Autodesk Inventor part; units mm, degrees
ref_plane "YZ Plane" through (0, 0, 0) normal (1, 0, 0) x (0, 1, 0)
ref_plane "XZ Plane" through (0, 0, 0) normal (0, 1, 0) x (-1, 0, 0)
ref_plane "XY Plane" through (0, 0, 0) normal (0, 0, 1) x (1, 0, 0)
sketch "Base" plane through (0, 0, 0) normal (0, 0, 1) x (1, 0, 0)
  line L0 (0, 0) -> (-33.5334, -57.9479)
  line L1 (22.7363, 2.3748) -> (0, 0)
  line L2 (68.7163, -13.2577) -> (22.7363, 2.3748)
  line L3 (-33.5334, -57.9479) -> (-26.9158, -67.5067)
  line L4 (-26.9158, -67.5067) -> (-51.547, -128.5125)
  line L5 (-51.547, -128.5125) -> (-33.4114, -135.8348)
  line L6 (-26.9158, -67.5067) -> (12.6221, -101.6388) construction
  line L7 (12.6221, -101.6388) -> (22.7363, -101.0656)
  line L8 (12.6221, -101.6388) -> (-8.1441, -124.1457)
  line L9 (-33.4114, -135.8348) -> (-8.1441, -124.1457)
  line L10 (22.7363, 2.3748) -> (68.7163, -13.2577)
  line L11 (68.7163, -13.2577) -> (112.7039, -111.8391)
  line L12 (22.7363, 2.3748) -> (22.7363, -101.0656) construction
  line L13 (22.7363, -101.0656) -> (65.9464, -171.4033)
  line L14 (112.7039, -111.8391) -> (105.2475, -122.1197)
  line L15 (22.7363, -101.0656) -> (112.7039, -111.8391) construction
  line L16 (105.2475, -122.1197) -> (103.571, -134.8197)
  line L17 (103.571, -134.8197) -> (108.4402, -146.5492)
  line L18 (65.9464, -171.4033) -> (74.9694, -180.3406)
  line L19 (108.4402, -146.5492) -> (74.9694, -180.3406)
  circle A0 centre (85.3652, -157.1655) radius 25.4
  line L20 (-42.4792, -132.1736) -> (22.7363, -49.3454) construction
  line L21 (-33.0514, -120.1997) -> (-25.1949, -110.2215) construction
  line L22 (-35.546, -118.2356) -> (-27.6895, -108.2573)
  line L23 (-22.7004, -112.1856) -> (-30.5568, -122.1638)
  arc A1 (-35.546, -118.2356) -> (-30.5568, -122.1638) centre (-33.0514, -120.1997) ccw
  arc A2 (-22.7004, -112.1856) -> (-27.6895, -108.2573) centre (-25.1949, -110.2215) ccw
  circle A3 centre (85.3652, -157.1655) radius 4
  line L24 (0, -219.5535) -> (0, 39.3628)
  point P0 (-29.1232, -115.2106)
  point P1 (60.5618, -162.6381)
  dimension "d4" = 50.8
  dimension "d5" = 22.86
  dimension "d6" = 155.26
  dimension "d7" = 126.02
  dimension "d8" = 48.5647
  dimension "d9" = 66.9511
  dimension "d10" = 132.824
  dimension "d11" = 107.95
  dimension "d12" = 115.248
  dimension "d13" = 11.6259
  dimension "d14" = 65.7906
  dimension "d15" = 19.558
  dimension "d16" = 120
  dimension "d17" = 12.7
  dimension "d18" = 12.7
  dimension "d19" = 12.7
  dimension "d20" = 82.55
  dimension "d21" = 12.7
  dimension "d24" = 15.24
  dimension "d26" = 12.7
  dimension "d31" = 8
  dimension "d32" = 95.963
  dimension "d33" = 38.215
  dimension "d34" = 22.545
  dimension "d35" = 7.52
  dimension "d36" = 44.727
  dimension "d37" = 31.563
  dimension "d38" = 86.757
  dimension "d39" = 42.697
  dimension "d40" = 49.197
  dimension "d41" = 114.826
  dimension "d47" = 105.4209
  dimension "d48" = 62.051
  dimension "d75" = 3.175
extrude "Plate1" add sketch "Base" along normal blind 5
fillet "OutsideFilletsFeature" radius 6.35 14 edges at (68.7163, -13.2577, 2.5) (22.7363, 2.3748, 2.5) (0, 0, 2.5) (-33.5334, -57.9479, 2.5) (-26.9158, -67.5067, 2.5) (-51.547, -128.5125, 2.5) (-33.4114, -135.8348, 2.5) (-8.1441, -124.1457, 2.5) (12.6221, -101.6388, 2.5) (22.7363, -101.0656, 2.5) (60.5618, -162.6381, 2.5) (103.571, -134.8197, 2.5) (105.2475, -122.1197, 2.5) (112.7039, -111.8391, 2.5)
sketch "MountHoles" plane through (0, 0, 5) normal (0, 0, 1) x (1, 0, 0)
  line L0 (-1.6199, -2.7989) -> (-30.9807, -53.5288) construction
  arc A0 (3.2163, 0.3359) -> (-1.6199, -2.7989) centre (3.876, -5.9797) ccw construction
  line L1 (21.3511, 2.2301) -> (3.2163, 0.3359) construction
  arc A1 (24.0549, 1.9264) -> (21.3511, 2.2301) centre (22.0108, -4.0856) ccw construction
  arc A2 (69.8461, -15.7897) -> (66.0912, -12.3652) centre (64.0472, -18.3772) ccw construction
  line L2 (24.0548, 1.9265) -> (66.0912, -12.3652) construction
  line L3 (66.0912, -12.3652) -> (24.0548, 1.9265) construction
  line L4 (-20.7142, -54.4632) -> (5.7075, -8.8047) construction
  line L5 (5.7075, -8.8047) -> (21.6681, -7.1377) construction
  line L6 (21.6681, -7.1377) -> (66.0912, -22.2408) construction
  line L7 (-31.5169, -54.4632) -> (-1.6198, -2.7992) construction
  line L8 (3.2166, 0.336) -> (21.3512, 2.2301) construction
  line L9 (24.0548, 1.9265) -> (66.0912, -12.3652) construction
  line L10 (-31.5169, -54.4632) -> (-20.7142, -54.4632) construction
  line L11 (66.0912, -22.2408) -> (66.0912, -12.3652) construction
  circle A3 centre (5.7075, -8.8047) radius 3
  circle A4 centre (21.6681, -7.1377) radius 3
  circle A5 centre (63.2509, -21.2751) radius 3
  point P0 (0, 0)
  dimension "d49" = 9.35
  dimension "d50" = 9.35
  dimension "d51" = 9.35
  dimension "d52" = 6
  dimension "d53" = 6
  dimension "d54" = 6
  dimension "d55" = 3
extrude "MountHolesFeature" cut sketch "MountHoles" against normal blind 5
equation "\"d50\" = d49"
equation "\"d51\" = d49"
equation "\"d56\" = Thickness"
equation "\"d42\" = Thickness"
equation "\"BendRadius\" = Thickness"
equation "\"BendReliefWidth\" = Thickness"
equation "\"BendReliefDepth\" = 0.5 * Thickness"
equation "\"TransitionRadius\" = BendRadius"
equation "\"JacobiRadiusSize\" = BendRadius"
equation "\"GapSize\" = Thickness"
properties part number "Knee"
Can you work these out from the model? Positions are in its coordinate system, mm. A direction names the side the tool comes from. Coordinates: 2 decimals unless noted, no trailing zeros. Loops run counter-clockwise (first coordinate to the right, second up) from the corner with the lowest first, then second, coordinate; pieces in that order, holes last. Notation, with made-up numbers: (-33.5, 49.25) -> (5.5, 49.25) arc R11 ccw to (5.5, 58.25) -> close; hole circle Ø7 at (-11.75, 70). An arc over 180 degrees is marked (long way). Put each result on its own line as item: value. Start each with the question number.
Q1. I want a section at A-A (x = 53.5). Write out the boundary of the cut face in (y, z), plus the area to 3 significant figures.
Q2. I want a section at B-B (z = 2.2). Count the separate pieces of the cut face and the enclosed holes in it, plus the area to 3 significant figures.
Q3. For faces 1 (the face through (90.24, -61.49, 2.46)), 2 (the face through (22.294, -102.015, 2.535)), 3 (the face through (104.424, -128.356, 2.465)), 4 (the face through (-26.57, -117.1, 2.46)), 5 (the face through (-49.153, -127.42, 2.535)), which set-ups out of +Z, -Z, +X, -X, +Y, -Y let a thin tool reach every point of the face, with its end or its side?
Q4. I want a section at C-C (y = -42). Write out the boundary of the cut face in (x, z), plus the area to 3 significant figures.
Q5. If I drill on line 1 (Y direction, x = -31.5, z = 1.85); line 2 (X direction, y = -132.5, z = 0.35); line 3 (Y direction, x = 3.5, z = 2.55), over which ranges is the centre line in solid material (lowest first)? Write a range as [from, to].
Q6. Thinking about a two-plate mould opening in X: for faces 6 (the face through (68.35, -13.71, 2.54)), 7 (the face through (-32.367, -57.85, 2.535)), 8 (the face through (8.569, -7.904, 2.535)), 9 (the face through (42.13, -132.635, 2.465)), which applies, pulls with the +X half, pulls with the -X half, needs draft (parallel to the pull), parting line crosses it, or undercut?
Taken from the geometry:
1. outline: (-151.14, 0) -> (-8.08, 0) -> (-8.08, 5) -> (-151.14, 5) -> close
1. area: 715 mm2
2. separate pieces: 1
2. enclosed holes: 5
2. area: 16,800 mm2
3. face 1: +Z, -Z, +X, +Y
3. face 2: +Z, -Z, -Y
3. face 3: +Z, -Z, +X
3. face 4: +Z, -Z
3. face 5: +Z, -Z, -X
4. outline: (-24.3, 0) -> (81.54, 0) -> (81.54, 5) -> (-24.3, 5) -> close
4. area: 529 mm2
5. line 1: y = [-134.92, -122.97], [-113.1, -78.86], [-60.85, -54.43]
5. line 2: x = [-41.67, -26.2], [42.05, 103.88]
5. line 3: y = [-111.53, -10.84], [-6.77, 0.37]
6. face 6: pulls with the +X half
6. face 7: pulls with the -X half
6. face 8: undercut
6. face 9: undercut
